Can you work these out from the drawing? Everything is in mm from the part's minimum corner. A direction names the side the tool comes from. Coordinates: 2 decimals unless noted, no trailing zeros. Order: outer loops, then holes, each group sorted by start corner. A loop starts at its lowest first (then second) coordinate and runs counter-clockwise, first axis right, second up. Notation, with made-up numbers: M -26.75,0 L 4.25,0 A14 cw 4.25,7 Z; hole C 53,46 d4. An arc over 180 degrees is marked long. One line per question, with ' | ' between items. Start each with the question number.
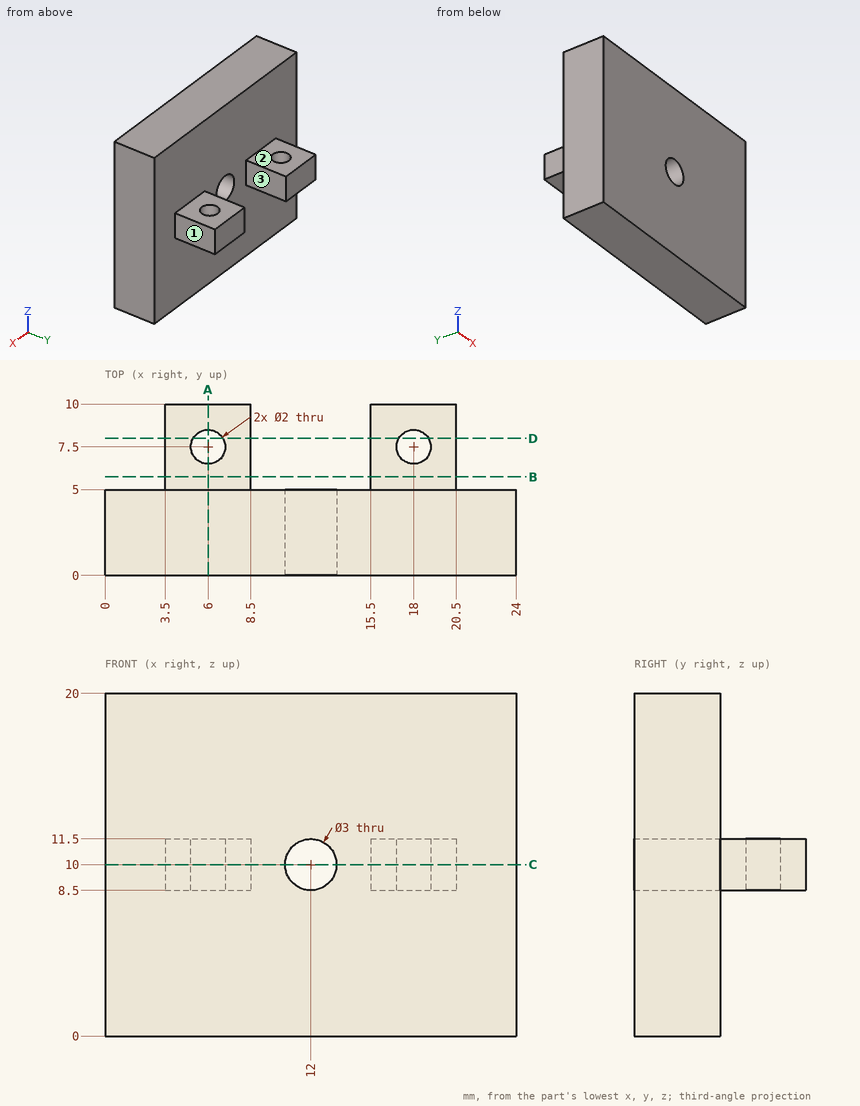
(1) For P1, Ø5.5, axis at x = 5, y = 8, coming from the -Z side; P2, Ø1.5, axis at y = 7.5, z = 9.5, coming from the +X side; P3, Ø1.5, axis at y = 6, z = 14, coming from the -X side; P4, Ø5.5, axis at x = 19, y = 8, coming from the +Z side, each with a flat end and sliding along its axis, tell me the tip position at first contact or that it passes through.
(2) Imagine slicing it at D-D, the plane y = 8. Write out the boundary of the cut face in (x, z), plus the area to 3 significant figures.
(3) Imagine slicing it at C-C, the plane z = 10. Write out the boundary of the cut face in (x, y), plus the area to 3 significant figures.
(4) Imagine slicing it at B-B, the plane y = 5.75. Write out the boundary of the cut face in (x, z).
(5) If I drill on line 1 along Y through (x, z) = (6, 10.05); line 2 along Z through (x, y) = (8.25, 5.25); line 3 along Y through (x, z) = (3.5, 4.75), over which ranges is the centre line in solid material (lowest first)? Write a range as from..to.
(6) Imagine slicing it at A-A, the plane x = 6. Write out the boundary of the cut face in (y, z), plus the area to 3 significant figures.
(7) On a 3-axis mill with a long thin cutter (end or side, diameter ignored), from which of +Z, -Z, +X, -X, +Y, -Y can I reach the whole of each face in a straight line? I mean the marked faces 1, 2 and 3. Say none if no direction works.
Answers:
1) P1: z = 8.5 | P2: x = 20.5 | P3: through | P4: z = 11.5
2) outline: M 3.5,8.5 L 5.13,8.5 L 5.13,11.5 L 3.5,11.5 Z; M 6.87,8.5 L 8.5,8.5 L 8.5,11.5 L 6.87,11.5 Z; M 15.5,8.5 L 17.13,8.5 L 17.13,11.5 L 15.5,11.5 Z; M 18.87,8.5 L 20.5,8.5 L 20.5,11.5 L 18.87,11.5 Z | area: 19.6 mm²
3) outline: M 0,0 L 10.5,0 L 10.5,5 L 8.5,5 L 8.5,10 L 3.5,10 L 3.5,5 L 0,5 Z; M 13.5,0 L 24,0 L 24,5 L 20.5,5 L 20.5,10 L 15.5,10 L 15.5,5 L 13.5,5 Z; hole C 6,7.5 d2; hole C 18,7.5 d2 | area: 149 mm²
4) outline: M 3.5,8.5 L 8.5,8.5 L 8.5,11.5 L 3.5,11.5 Z; M 15.5,8.5 L 20.5,8.5 L 20.5,11.5 L 15.5,11.5 Z
5) line 1: 0..6.5, 8.5..10 | line 2: 8.5..11.5 | line 3: 0..5
6) outline: M 0,0 L 5,0 L 5,8.5 L 6.5,8.5 L 6.5,11.5 L 5,11.5 L 5,20 L 0,20 Z; M 8.5,8.5 L 10,8.5 L 10,11.5 L 8.5,11.5 Z | area: 109 mm²
7) face 1: +Z, -Z, +X, +Y | face 2: +Z, +X, -X, +Y | face 3: +Z, -Z, +Y
